Part model, mm, in its own coordinate system. A direction names the side the tool comes from. Coordinates: 2 decimals unless noted, no trailing zeros. Loops run counter-clockwise (first coordinate to the right, second up) from the corner with the lowest first, then second, coordinate; pieces in that order, holes last.
```python
from build123d import *
from build123d.topology import SkipClean

# Parameters (mm, degrees)
EXTRUDE_1_DEPTH     = 1
EXTRUDE_2_DEPTH     = 1.4
EXTRUDE_3_DEPTH     = 2.4
CUT_EXTRUDE_2_REACH = 134.888
SKETCH_4_R          = 1.7
CUT_EXTRUDE_3_DEPTH = 10
CUT_EXTRUDE_4_REACH = 134.874
SKETCH_6_W          = 6.2
SKETCH_6_H          = 0.2
FILLET_START        = -1.2
FILLET_1_DEPTH      = 2.2
FILLET_START_2      = -1.4
FILLET_1_2_DEPTH    = 0.226512
SKETCH_7_W          = 9
SKETCH_7_H          = 2.5
CUT_EXTRUDE_5_DEPTH = 133.88811083
EXTRUDE_4_REACH     = 113.48


with BuildPart() as part:
    # 草图1 → 凸台-拉伸1 (new body)
    with BuildSketch(Plane(origin=(0, 0, 0), x_dir=(1, 0, 0), z_dir=(0, 1, 0))):
        Polygon((0, 0), (12.75, 94), (76.75, 94), (89.5, 0), align=None)
    extrude(amount=EXTRUDE_1_DEPTH)

    # 草图2 → 凸台-拉伸2 (add)
    with BuildSketch(Plane.XZ):
        Polygon((89.5, 0), (0, 0), (12.75, -94), (76.75, -94), align=None)
        Polygon((87.897286654, -1.4), (1.602713346, -1.4), (13.972926112, -92.6), (75.527073888, -92.6), align=None, mode=Mode.SUBTRACT)
    extrude(amount=EXTRUDE_2_DEPTH)

    # 草图3 → 凸台-拉伸3 (add)
    with BuildSketch(Plane(origin=(0, 1, 0), x_dir=(1, 0, 0), z_dir=(0, 1, 0))):
        with BuildLine():
            Line((6.25, -1.2), (6.25, 0))
            Line((6.25, 0), (8.545840542, 0))
            ThreePointArc((8.545840542, 0), (9.75, -2.9), (10.954159458, 0))
            Line((10.954159458, 0), (13.25, 0))
            Line((13.25, 0), (13.25, -1.2))
            ThreePointArc((13.25, -1.2), (9.75, -4.7), (6.25, -1.2))
        make_face()
        with BuildLine():
            Line((13.75, 94.7), (13.75, 94))
            Line((13.75, 94), (13.82071436, 94))
            Line((13.82071436, 94), (15.700806662, 94))
            ThreePointArc((15.700806662, 94), (17.25, 96.4), (18.799193338, 94))
            Line((18.799193338, 94), (20.75, 94))
            Line((20.75, 94), (20.75, 94.7))
            ThreePointArc((20.75, 94.7), (17.25, 98.2), (13.75, 94.7))
        make_face()
        with BuildLine():
            Line((68.75, 94.7), (68.75, 94))
            Line((68.75, 94), (70.700806662, 94))
            ThreePointArc((70.700806662, 94), (72.25, 96.4), (73.799193338, 94))
            Line((73.799193338, 94), (75.75, 94))
            Line((75.75, 94), (75.75, 94.7))
            ThreePointArc((75.75, 94.7), (72.25, 98.2), (68.75, 94.7))
        make_face()
    extrude(amount=-EXTRUDE_3_DEPTH)

    # 草图4 → 切除-拉伸2 (cut, up to next)
    with BuildSketch(Plane(origin=(0, 1, 0), x_dir=(1, 0, 0), z_dir=(0, 1, 0)), mode=Mode.PRIVATE) as cut_extrude_2_sk1:
        with Locations(Location((9.75, -1.2, 0), (0, 0, 270))):
            Circle(SKETCH_4_R)
    cut_extrude_2_tool1 = extrude(cut_extrude_2_sk1.sketch, amount=-CUT_EXTRUDE_2_REACH, mode=Mode.PRIVATE) & part.part
    # 草图4 → 切除-拉伸2 (cut, up to next)
    with BuildSketch(Plane(origin=(0, 1, 0), x_dir=(1, 0, 0), z_dir=(0, 1, 0)), mode=Mode.PRIVATE) as cut_extrude_2_sk2:
        with Locations(Location((17.25, 94.7, 0), (0, 0, 270))):
            Circle(SKETCH_4_R)
    cut_extrude_2_tool2 = extrude(cut_extrude_2_sk2.sketch, amount=-CUT_EXTRUDE_2_REACH, mode=Mode.PRIVATE) & part.part
    # 草图4 → 切除-拉伸2 (cut, up to next)
    with BuildSketch(Plane(origin=(0, 1, 0), x_dir=(1, 0, 0), z_dir=(0, 1, 0)), mode=Mode.PRIVATE) as cut_extrude_2_sk3:
        with Locations(Location((72.25, 94.7, 0), (0, 0, 270))):
            Circle(SKETCH_4_R)
    cut_extrude_2_tool3 = extrude(cut_extrude_2_sk3.sketch, amount=-CUT_EXTRUDE_2_REACH, mode=Mode.PRIVATE) & part.part
    add(cut_extrude_2_tool1.solids().sort_by_distance((9.75, 1, 1.2))[0], mode=Mode.SUBTRACT)
    add(cut_extrude_2_tool2.solids().sort_by_distance((17.25, 1, -94.7))[0], mode=Mode.SUBTRACT)
    add(cut_extrude_2_tool3.solids().sort_by_distance((72.25, 1, -94.7))[0], mode=Mode.SUBTRACT)

    # 草图5 → 切除-拉伸3 (cut)
    with SkipClean():  # the faces are left unmerged after this step: merging them gives an invalid solid
        with BuildSketch(Plane(origin=(0, 1, 0), x_dir=(1, 0, 0), z_dir=(0, 1, 0))):
            with BuildLine():
                Line((78.21236986, 90.741242548), (74.942313599, 90.297697683))
                Line((74.942313599, 90.297697683), (76.017573878, 82.370288564))
                Line((76.017573878, 82.370288564), (79.28763014, 82.81383343))
                ThreePointArc((79.28763014, 82.81383343), (82.713704559, 87.315168128), (78.21236986, 90.741242548))
            make_face()
            with BuildLine():
                Line((38.75, -1.222462011), (38.75, 2.277537989))
                Line((38.75, 2.277537989), (46.75, 2.277537989))
                Line((46.75, 2.277537989), (46.75, -1.222462011))
                ThreePointArc((46.75, -1.222462011), (42.75, -5.222462011), (38.75, -1.222462011))
            make_face()
            with BuildLine():
                Line((75.75, -1.222462011), (75.75, 2.277537989))
                Line((75.75, 2.277537989), (83.75, 2.277537989))
                Line((83.75, 2.277537989), (83.75, -1.222462011))
                ThreePointArc((83.75, -1.222462011), (79.75, -5.222462011), (75.75, -1.222462011))
            make_face()
        extrude(amount=-CUT_EXTRUDE_3_DEPTH, mode=Mode.SUBTRACT)

    # 草图6 → 切除-拉伸4 (cut, up to next)
    with BuildSketch(Plane(origin=(0, 0, 0), x_dir=(0, 0, -1), z_dir=(1, 0, 0)), mode=Mode.PRIVATE) as cut_extrude_4_sk1:
        with Locations((95.1, -1.3)):
            Rectangle(SKETCH_6_W, SKETCH_6_H)
    cut_extrude_4_tool1 = extrude(cut_extrude_4_sk1.sketch, amount=CUT_EXTRUDE_4_REACH, mode=Mode.PRIVATE) & part.part
    add(cut_extrude_4_tool1.solids().sort_by_distance((0, -1.3, -95.1))[0], mode=Mode.SUBTRACT)

    # 圆角1: read off the stored shape, not the designer's step
    # 圆角1 outline → 圆角1 (add)
    with SkipClean():  # the faces are left unmerged after this step: merging them gives an invalid solid
        with BuildSketch(Plane(origin=(0, 0, 0), x_dir=(1, 0, 0), z_dir=(0, 1, 0)).offset(FILLET_START)):
            with BuildLine():
                ThreePointArc((13.25, -1.2), (13.240681915, -1.455224942), (13.212777274, -1.709090909))
                ThreePointArc((13.212777274, -1.709090909), (13.884185107, -0.486425063), (15.191507144, 0))
                Line((15.191507144, 0), (13.25, 0))
                Line((13.25, 0), (13.25, -1.2))
            make_face()
            with BuildLine():
                ThreePointArc((4.308492856, 0), (5.615814893, -0.486425063), (6.287222726, -1.709090909))
                ThreePointArc((6.287222726, -1.709090909), (6.259318085, -1.455224942), (6.25, -1.2))
                Line((6.25, -1.2), (6.25, 0))
                Line((6.25, 0), (4.308492856, 0))
            make_face()
            with BuildLine():
                Line((75.75, 94), (76.75, 94))
                ThreePointArc((76.75, 94), (76.053957158, 94.573295448), (75.680491288, 95.394067374))
                ThreePointArc((75.680491288, 95.394067374), (75.732579469, 95.048769616), (75.75, 94.7))
                Line((75.75, 94.7), (75.75, 94))
            make_face()
            with BuildLine():
                ThreePointArc((13.75, 94.7), (13.767420531, 95.048769616), (13.819508712, 95.394067374))
                ThreePointArc((13.819508712, 95.394067374), (13.446042842, 94.573295448), (12.75, 94))
                Line((12.75, 94), (13.75, 94))
                Line((13.75, 94), (13.75, 94.7))
            make_face()
            with BuildLine():
                Line((20.75, 94), (22.594155686, 94))
                ThreePointArc((22.594155686, 94), (21.358326925, 94.427509214), (20.650826346, 95.527272727))
                ThreePointArc((20.650826346, 95.527272727), (20.725118143, 95.116598001), (20.75, 94.7))
                Line((20.75, 94.7), (20.75, 94))
            make_face()
            with BuildLine():
                ThreePointArc((68.75, 94.7), (68.774881857, 95.116598001), (68.849173654, 95.527272727))
                ThreePointArc((68.849173654, 95.527272727), (68.141673075, 94.427509214), (66.905844314, 94))
                Line((66.905844314, 94), (68.75, 94))
                Line((68.75, 94), (68.75, 94.7))
            make_face()
        extrude(amount=FILLET_1_DEPTH)

    # Fillet 1 2 outline → Fillet 1 2 (add)
    with SkipClean():  # the faces are left unmerged after this step: merging them gives an invalid solid
        with BuildSketch(Plane(origin=(0, 0, 0), x_dir=(1, 0, 0), z_dir=(0, 1, 0)).offset(FILLET_START_2)):
            with BuildLine():
                ThreePointArc((13.25, -1.2), (13.240681915, -1.455224942), (13.212777274, -1.709090909))
                ThreePointArc((13.212777274, -1.709090909), (13.884185107, -0.486425063), (15.191507144, 0))
                Line((15.191507144, 0), (13.25, 0))
                Line((13.25, 0), (13.25, -1.2))
            make_face()
            with BuildLine():
                ThreePointArc((4.308492856, 0), (5.615814893, -0.486425063), (6.287222726, -1.709090909))
                ThreePointArc((6.287222726, -1.709090909), (6.259318085, -1.455224942), (6.25, -1.2))
                Line((6.25, -1.2), (6.25, 0))
                Line((6.25, 0), (4.308492856, 0))
            make_face()
        extrude(amount=FILLET_1_2_DEPTH)

    # 草图7 → 切除-拉伸5 (cut, through all)
    with SkipClean():  # the faces are left unmerged after this step: merging them gives an invalid solid
        with BuildSketch(Plane(origin=(0, 1, 0), x_dir=(1, 0, 0), z_dir=(0, 1, 0))):
            with Locations((32.25, 1.25)):
                Rectangle(SKETCH_7_W, SKETCH_7_H)
        extrude(amount=-CUT_EXTRUDE_5_DEPTH, mode=Mode.SUBTRACT)

    # 草图8 → 凸台-拉伸4 (add, up to next)
    with BuildSketch(Plane.ZY.offset(-36.75), mode=Mode.PRIVATE) as extrude_4_sk1:
        Polygon((-2.5, 0.653445531), (-1.819327572, 0), (-2.5, 0), align=None)
    extrude_4_tool1 = extrude(extrude_4_sk1.sketch, amount=EXTRUDE_4_REACH, mode=Mode.PRIVATE) - part.part
    # 草图8 → 凸台-拉伸4 (add, up to next)
    with BuildSketch(Plane.ZY.offset(-36.75), mode=Mode.PRIVATE) as extrude_4_sk2:
        Polygon((-0.360994239, -1.4), (-1.4, -1.4), (-1.4, -0.402554469), align=None)
    extrude_4_tool2 = extrude(extrude_4_sk2.sketch, amount=EXTRUDE_4_REACH, mode=Mode.PRIVATE) - part.part
    add(extrude_4_tool1.solids().sort_by_distance((36.75, 0.217815, -2.273109))[0])
    add(extrude_4_tool2.solids().sort_by_distance((36.75, -1.067518, -1.053665))[0])


solid = part.part
```
Q1. Drop flat-ended pins along their axis: P1, Ø0.7, axis at x = 54, y = -1, coming from the -Z side; P2, Ø5, axis at x = 45, z = -95, coming from the -Y side; P3, Ø0.8, axis at x = 80.5, y = 0.5, coming from the +Z side. Give the stop position or say it passes through.
Q2. Saw through at B-B (x = 51.5). List the corners of the cut face in (y, z).
Q3. Saw through at C-C (z = -14.5). List the corners of the cut face in (x, y).
Q4. Mould opens along X. For faces 4 (the flat face through (6.286, -0.183, -46.342)), 5 (the flat face through (44, 0, -94)), 6 (the flat face through (45, 1, -47)) say: released by +X, released by -X, zero draft, split by the parting line, or undercut.
Q5. Tool access for faces 1 (the flat face through (61, 0, 0)), 2 (the flat face through (7.7, -0.69, -46.36)), 3 (the flat face through (44.6, -1.2, -93.7)): list every direction of +Z, -Z, +X, -X, +Y, -Y with a clear straight run to the whole face (end or side of a thin tool).
Q6. Saw through at D-D (x = 9.75). List the corners of the cut face in (y, z).
Q7. Saw through at A-A (x = 72.25). List the corners of the cut face in (y, z).
Q8. Probe line 1 (Z direction, x = 54, y = -0.4); line 2 (X direction, y = -0.2, z = -94.7); line 3 (Y direction, x = 73.5, z = -88). List the from-to ranges inside material, lowest first.
Checked values:
1. P1: stops at z = -94
1. P2: stops at y = -1.2
1. P3: stops at z = -2.28
2. outline: (-1.4, -1.4) - (0, -1.4) - (0, -92.6) - (-1.2, -92.6) - (-1.2, -94) - (1, -94) - (1, 0) - (-1.4, 0) - close
3. outline: (1.97, -1.4) - (3.38, -1.4) - (3.38, 0) - (86.12, 0) - (86.12, -1.4) - (87.53, -1.4) - (87.53, 1) - (1.97, 1) - close
4. face 4: released by -X
4. face 5: undercut
4. face 6: zero draft
5. face 1: +Z, +X, +Y, -Y
5. face 2: -Y
5. face 3: -Z, +X, -X, -Y
6. outline: (-1.4, -71.88) - (1, -71.88) - (1, -0.5) - (-1.4, -0.5) - (-1.4, -1.4) - (0, -1.4) - (0, -61.47) - (-1.4, -61.47) - close; (-1.4, 2.9) - (1, 2.9) - (1, 4.7) - (-1.4, 4.7) - close
7. outline: (-1.4, -1.4) - (0, -1.4) - (0, -92.6) - (-1.2, -92.6) - (-1.2, -93) - (1, -93) - (1, 0) - (-1.4, 0) - close; (-1.2, -98.2) - (1, -98.2) - (1, -96.4) - (-1.2, -96.4) - close
8. line 1: z = -94 to -92.6, -1.4 to 0
8. line 2: x = 13.54 to 15.55, 18.95 to 21.07, 68.43 to 70.55, 73.95 to 75.96
8. line 3: y = 0 to 1
